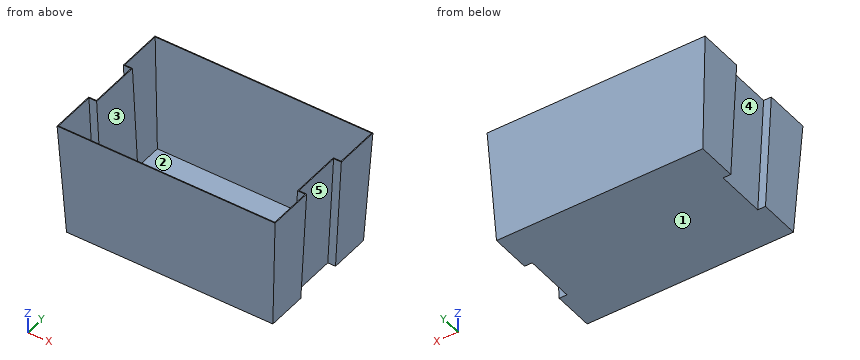
```python
from build123d import *

# Parameters (mm, degrees)
F4_T = 2


with BuildPart() as f3:
    # F0 (on Top) → F3 section 0
    with BuildSketch(Plane.XY):
        Polygon((252.4125, 158.75), (-252.4125, 158.75), (-252.4125, 63.5), (-233.3625, 63.5), (-233.3625, -63.5), (-252.4125, -63.5), (-252.4125, -158.75), (252.4125, -158.75), (252.4125, -63.5), (233.3625, -63.5), (233.3625, 63.5), (252.4125, 63.5), align=None)
    # F2 (on offset) → F3 section 1
    with BuildSketch(Plane.XY.offset(279.4)):
        Polygon((266.7, 171.45), (-266.7, 171.45), (-266.7, 63.5), (-247.65, 63.5), (-247.65, -63.5), (-266.7, -63.5), (-266.7, -171.45), (266.7, -171.45), (266.7, -63.5), (247.65, -63.5), (247.65, 63.5), (266.7, 63.5), align=None)
    loft()

    # F4
    f4_openings = [f3.faces().sort_by_distance(p)[0] for p in [
        (0, 0, 279.4),
    ]]
    offset(amount=F4_T, openings=f4_openings, kind=Kind.INTERSECTION)


solid = f3.part
```
For this review, take the finished solid that the model builds, in its own axes (mm). Face numbers are marked on the shaded views. A direction names the side the tool comes from. Give positions to 0.01 mm unless a question says otherwise; leave off trailing zeros. Write each loop counter-clockwise with the first axis right and the second up, starting at its lowest first coordinate (ties: lowest second). Pieces come first, ordered by that corner, then holes.
Item 1: Take a section at A-A (y = 39). Give the boundary of the cut face in (x, z), and give its area (3 significant figures).
Item 2: The part is to be moulded in two halves that separate along Y. For the marked faces 1, 2 and 3, say which applies: +Y half, -Y half, draft (parallel to the pull), parting line (faces both ways), or undercut.
Item 3: Insertion check: P1, Ø3, axis at y = 48, z = 107, coming from the -X side; P2, Ø5, axis at x = 101, z = 177, coming from the -Y side; P3, Ø4, axis at x = -183.5, z = 232, coming from the +Y side. Each pin has a flat end and moves straight along its axis. Give the tip position at first contact, or say it passes through.
Item 4: Wall thickness on probe 1 along Z at (x, y) = (185, -156); probe 2 along Y at (x, z) = (-91, 69); probe 3 along Y at (x, z) = (98, 230.5): over which ranges is each line inside the solid? List them lowest first.
Item 5: Machinability: for the marked faces 4 and 5, which of the approach directions +Z, -Z, +X, -X, +Y, -Y give a long, thin tool a straight path to every point of the face, cutting with its end or side? Answer none if there is none.
Established:
1. outline: (-249.65, 279.4) - (-235.26, -2) - (235.26, -2) - (249.65, 279.4) - (247.65, 279.4) - (233.36, 0) - (-233.36, 0) - (-247.65, 279.4) - close
1. area: 2,060 mm2
2. face 1: draft
2. face 2: undercut
2. face 3: undercut
3. P1: stops at x = -240.91
3. P2: stops at y = -168.91
3. P3: stops at y = 171.39
4. probe 1: z = -2 to 0
4. probe 2: y = -163.89 to -161.89, 161.89 to 163.89
4. probe 3: y = -171.23 to -169.23, 169.23 to 171.23
5. face 4: -Z, -X
5. face 5: -Z, +X
